```python
from build123d import *

# Parameters (mm, degrees)
SKETCH1_W           = 60
SKETCH1_H           = 62.5
BOSS_EXTRUDE1_DEPTH = 3
SKETCH2_W           = 60
SKETCH2_H           = 64.2
BOSS_EXTRUDE2_DEPTH = 3
FILLET1_RADIUS      = 30
FILLET1_LENGTH      = 3
SKETCH3_R           = 16.5
SKETCH3_R_2         = 2.6
CUT_EXTRUDE1_DEPTH  = 3


with BuildPart() as part:
    # Sketch1 → Boss-Extrude1 (new body)
    with BuildSketch(Plane.XY):
        with Locations((30, 31.25)):
            Rectangle(SKETCH1_W, SKETCH1_H)
        with BuildLine():
            Line((7.8, 10.1), (7.8, 52.4))
            ThreePointArc((7.8, 52.4), (9.8, 54.4), (11.8, 52.4))
            Line((11.8, 52.4), (11.8, 10.1))
            ThreePointArc((11.8, 10.1), (9.8, 8.1), (7.8, 10.1))
        make_face(mode=Mode.SUBTRACT)
        with BuildLine():
            Line((48.2, 10.1), (48.2, 52.4))
            ThreePointArc((48.2, 52.4), (50.2, 54.4), (52.2, 52.4))
            Line((52.2, 52.4), (52.2, 10.1))
            ThreePointArc((52.2, 10.1), (50.2, 8.1), (48.2, 10.1))
        make_face(mode=Mode.SUBTRACT)
    extrude(amount=BOSS_EXTRUDE1_DEPTH)

    # Sketch2 → Boss-Extrude2 (add)
    with BuildSketch(Plane(origin=(0, 62.5, 0), x_dir=(1, 0, 0), z_dir=(0, 1, 0))):
        with Locations((30, 29.1)):
            Rectangle(SKETCH2_W, SKETCH2_H)
    extrude(amount=-BOSS_EXTRUDE2_DEPTH)

    # Fillet1: full round fillet: the end face becomes a half cylinder, R = half its width
    fillet1_face = Plane((30, 61, -61.2), x_dir=(0, 1, 0), z_dir=(0, 0, -1))  # on the end face: x along it, z out of the body
    fillet1_slab = fillet1_face.offset(-FILLET1_RADIUS / 2) * Box(FILLET1_LENGTH, 2 * FILLET1_RADIUS, FILLET1_RADIUS, mode=Mode.PRIVATE)  # the body's end, R deep
    fillet1_round = Plane((30, 61, -31.2), x_dir=(0, 0, -1), z_dir=(0, 1, 0)) * Cylinder(FILLET1_RADIUS, FILLET1_LENGTH, mode=Mode.PRIVATE)  # its axis R under the face
    add(fillet1_slab - fillet1_round, mode=Mode.SUBTRACT)

    # Sketch3 → Cut-Extrude1 (cut)
    with BuildSketch(Plane(origin=(0, 62.5, 0), x_dir=(1, 0, 0), z_dir=(0, 1, 0))):
        with Locations(Location((30, 31.2, 0), (0, 0, 270))):
            Circle(SKETCH3_R)
        with Locations(Location((30, 52.2, 0), (0, 0, 270))):
            Circle(SKETCH3_R_2)
        with Locations(Location((51, 31.2, 0), (0, 0, 270))):
            Circle(SKETCH3_R_2)
        with Locations(Location((30, 10.2, 0), (0, 0, 270))):
            Circle(SKETCH3_R_2)
        with Locations(Location((9, 31.2, 0), (0, 0, 270))):
            Circle(SKETCH3_R_2)
    extrude(amount=-CUT_EXTRUDE1_DEPTH, mode=Mode.SUBTRACT)


solid = part.part
```
For this review, take the finished solid that the model builds, in its own axes (mm). A direction names the side the tool comes from. Give positions to 0.01 mm unless a question says otherwise; leave off trailing zeros. Write each loop counter-clockwise with the first axis right and the second up, starting at its lowest first coordinate (ties: lowest second). Pieces come first, ordered by that corner, then holes.
Item 1: The part is to be moulded in two halves that separate along Z. For faces 1 (the face through (30.66, 61.021, -61.193)), 2 (the face through (9.8, 8.1, 1.5)), 3 (the face through (32.19, 61.02, -8.8)), say which applies: +Z half, -Z half, draft (parallel to the pull), parting line (faces both ways), or undercut.
Item 2: Take a section at C-C (x = 30). Give the boundary of the cut face in (y, z).
Item 3: Take a section at A-A (y = 27.5). Give the boundary of the cut face in (x, z).
Item 4: Machinability: for faces 4 (the face through (30, 30, 0)), 5 (the face through (60, 40, 1)), 6 (the face through (50.2, 54.4, 1.5)), which of the approach directions +Z, -Z, +X, -X, +Y, -Y give a long, thin tool a straight path to every point of the face, cutting with its end or side? Answer none if there is none.
Item 5: Take a section at D-D (x = 41). Give the boundary of the cut face in (y, z).
Item 6: Take a section at B-B (z = -10.2). Give the boundary of the cut face in (x, y), and give its area (3 significant figures).
Item 7: Insertion check: P1, Ø3, axis at x = 40, y = 25, coming from the -Z side; P2, Ø4.5, axis at x = 51, z = -31.2, coming from the +Y side; P3, Ø2, axis at x = 47.5, z = -14.5, coming from the -Y side. Each pin has a flat end and moves straight along its axis. Give the tip position at first contact, or say it passes through.
Item 8: Wall thickness on probe 1 along X at (y, z) = (61, -31); probe 2 along Y at (x, z) = (6, -21.5); probe 3 along Z at (x, y) = (27.5, 17): over which ranges is each line inside the solid? List them lowest first.
Established:
1. face 1: -Z half
1. face 2: draft
1. face 3: undercut
2. outline: (0, 0) - (59.5, 0) - (59.5, -7.6) - (62.5, -7.6) - (62.5, 3) - (0, 3) - close; (59.5, -61.2) - (62.5, -61.2) - (62.5, -54.8) - (59.5, -54.8) - close; (59.5, -49.6) - (62.5, -49.6) - (62.5, -47.7) - (59.5, -47.7) - close; (59.5, -14.7) - (62.5, -14.7) - (62.5, -12.8) - (59.5, -12.8) - close
3. outline: (0, 0) - (7.8, 0) - (7.8, 3) - (0, 3) - close; (11.8, 0) - (48.2, 0) - (48.2, 3) - (11.8, 3) - close; (52.2, 0) - (60, 0) - (60, 3) - (52.2, 3) - close
4. face 4: -Z, +X, -X, -Y
4. face 5: +Z, -Z, +X, +Y, -Y
4. face 6: +Z, -Z
5. outline: (0, 0) - (59.5, 0) - (59.5, -18.9) - (62.5, -18.9) - (62.5, 3) - (0, 3) - close; (59.5, -59.11) - (62.5, -59.11) - (62.5, -43.5) - (59.5, -43.5) - close
6. outline: (0, 59.5) - (27.4, 59.5) - (27.4, 62.5) - (0, 62.5) - close; (32.6, 59.5) - (60, 59.5) - (60, 62.5) - (32.6, 62.5) - close
6. area: 164 mm2
7. P1: stops at z = 0
7. P2: passes through
7. P3: stops at y = 59.5
8. probe 1: x = 0 to 6.41, 11.59 to 13.5, 46.5 to 48.41, 53.59 to 60
8. probe 2: y = 59.5 to 62.5
8. probe 3: z = 0 to 3
